Input: part model. Units: mm. Frame: model coordinates. A direction names the side the tool comes from. Coordinates: 2 decimals unless noted, no trailing zeros. Write each loop counter-clockwise with the first axis right and the second up, starting at its lowest first coordinate (ties: lowest second). Pieces come first, ordered by that corner, then holes. Notation, with made-up numbers: (49.5, 29) - (108.5, 29) arc R17 ccw to (108.5, 51) - close; hole circle Ø1 at (47, -15.75). An arc over 180 degrees is marked (long way). Use a Markdown table: item, result. Add a question column.
Q1. Section query C-C (z = 2.5). Give the number of separate pieces and of enclosed holes in the cut face, then the cut area to 3 significant figures.
Q2. Mould query, pull axis Y, two halves, no side actions, for faces 1 (the face through (72, 42, 0)), 2 (the face through (-95.47, -101.99, 1.57)), 3 (the face through (124.424, 125.214, 1.61)), 4 (the face through (-31.2, 16.3, 0.8)). Classes: released by +Y, released by -Y, zero draft, split by the parting line, or undercut.
Q3. Section query A-A (y = 39). Return the cut outline in (x, z) (1 decimal), then the cut area to 3 significant figures.
Q4. Pin query (flat end, axial travel): P1, Ø1.5, axis at x = 40, z = 2, coming from the -Y side; P2, Ø1, axis at y = 28.5, z = 2, coming from the -X side; P3, Ø1.5, axis at y = 15.5, z = 1, coming from the -X side. Return the tip coordinate at first contact, or that it passes through.
Q5. Set-up query: faces 5 (the face through (-67, -31, 1.588)), 6 (the face through (-122.77, -32.16, 1.61)). Return all of +Z, -Z, +X, -X, +Y, -Y with unobstructed straight access to the full face (end or side cutting, diameter ignored); none if empty.
Q6. Section query B-B (x = -116). Return the cut outline in (y, z) (1 decimal).
Q7. Section query D-D (y = -93.5). Return the cut outline in (x, z) (3 decimals).
Q8. Material intervals for probe 1 along X at (y, z) = (100, 0.7); probe 2 along Y at (x, z) = (60, 0.2); probe 3 along Y at (x, z) = (24.5, 2.35), sorted ascending. Write a range as from..to.
from build123d import *

# Parameters (mm, degrees)
BOSS_EXTRUDE1_DEPTH = 3.175
CUT_EXTRUDE3_DEPTH  = 1.5875
SKETCH3_R           = 9.525
CUT_EXTRUDE4_DEPTH  = 4.175
CUT_EXTRUDE5_DEPTH  = 4.175
FILLET1_R           = 50.8
SKETCH8_R           = 3.175
CUT_EXTRUDE7_DEPTH  = 4.175
SKETCH9_R           = 2.413
CUT_EXTRUDE8_DEPTH  = 4.175


with BuildPart() as part:
    # Sketch1 → Boss-Extrude1 (new body)
    with BuildSketch(Plane.XY):
        with BuildLine():
            Line((0, 139.7), (139.7, 139.7))
            Line((139.7, 139.7), (139.7, 0))
            ThreePointArc((139.7, 0), (-98.782817332, -98.782817332), (0, 139.7))
        make_face()
    extrude(amount=BOSS_EXTRUDE1_DEPTH)

    # Sketch2 → Cut-Extrude3 (cut)
    with BuildSketch(Plane(origin=(0, 0, 0), x_dir=(-1, 0, 0), z_dir=(0, 0, -1))):
        with BuildLine():
            ThreePointArc((-127.273929282, -57.597195461), (-126.611197849, -59.039771165), (-125.932116301, -60.474722685))
            Line((-125.932116301, -60.474722685), (-1.5875, -2.491875854))
            Line((-1.5875, -2.491875854), (-1.5875, -69.587590332))
            ThreePointArc((-1.5875, -69.587590332), (0, -69.162220989), (1.5875, -69.587590332))
            Line((1.5875, -69.587590332), (1.5875, -2.491875854))
            Line((1.5875, -2.491875854), (125.932116301, -60.474722685))
            ThreePointArc((125.932116301, -60.474722685), (126.611197849, -59.039771165), (127.273929282, -57.597195461))
            Line((127.273929282, -57.597195461), (3.756345013, 0))
            Line((3.756345013, 0), (55.328894815, 24.048674923))
            ThreePointArc((55.328894815, 24.048674923), (54.272472776, 25.307669683), (53.987081834, 26.926202147))
            Line((53.987081834, 26.926202147), (1.5875, 2.491875854))
            Line((1.5875, 2.491875854), (1.5875, 139.690979822))
            ThreePointArc((1.5875, 139.690979822), (0.793762813, 139.697744937), (0, 139.7))
            Line((0, 139.7), (-1.5875, 139.7))
            Line((-1.5875, 139.7), (-1.5875, 2.491875854))
            Line((-1.5875, 2.491875854), (-53.987081834, 26.926202147))
            ThreePointArc((-53.987081834, 26.926202147), (-54.272472776, 25.307669683), (-55.328894815, 24.048674923))
            Line((-55.328894815, 24.048674923), (-3.756345013, 0))
            Line((-3.756345013, 0), (-127.273929282, -57.597195461))
        make_face()
    extrude(amount=-CUT_EXTRUDE3_DEPTH, mode=Mode.SUBTRACT)

    # Sketch3 → Cut-Extrude4 (cut, through all)
    with BuildSketch(Plane.XY.offset(3.175)):
        Circle(SKETCH3_R)
    extrude(amount=-CUT_EXTRUDE4_DEPTH, mode=Mode.SUBTRACT)

    # Sketch2_4 → Cut-Extrude5 (cut, through all)
    with BuildSketch(Plane(origin=(0, 0, 0), x_dir=(-1, 0, 0), z_dir=(0, 0, -1))):
        with BuildLine():
            Line((-60.312918166, 26.37276318), (-55.328894815, 24.048674923))
            ThreePointArc((-55.328894815, 24.048674923), (-54.333740605, 25.183430817), (-53.975, 26.649482664))
            ThreePointArc((-53.975, 26.649482664), (-53.978021896, 26.787974218), (-53.987081834, 26.926202147))
            Line((-53.987081834, 26.926202147), (-58.971105185, 29.250290404))
            ThreePointArc((-58.971105185, 29.250290404), (-60.027527224, 27.991295645), (-60.312918166, 26.37276318))
        make_face()
        with BuildLine():
            ThreePointArc((-60.312918166, 26.37276318), (-58.491812981, 23.77195544), (-55.328894815, 24.048674923))
            Line((-55.328894815, 24.048674923), (-60.312918166, 26.37276318))
        make_face()
        with BuildLine():
            Line((-58.971105185, 29.250290404), (-53.987081834, 26.926202147))
            ThreePointArc((-53.987081834, 26.926202147), (-55.808187019, 29.527009887), (-58.971105185, 29.250290404))
        make_face()
        with BuildLine():
            ThreePointArc((53.987081834, 26.926202147), (54.272472776, 25.307669683), (55.328894815, 24.048674923))
            Line((55.328894815, 24.048674923), (60.312918166, 26.37276318))
            ThreePointArc((60.312918166, 26.37276318), (60.321978104, 26.510991109), (60.325, 26.649482664))
            ThreePointArc((60.325, 26.649482664), (59.966259395, 28.115534511), (58.971105185, 29.250290404))
            Line((58.971105185, 29.250290404), (53.987081834, 26.926202147))
        make_face()
        with BuildLine():
            ThreePointArc((58.971105185, 29.250290404), (55.808187019, 29.527009887), (53.987081834, 26.926202147))
            Line((53.987081834, 26.926202147), (58.971105185, 29.250290404))
        make_face()
        with BuildLine():
            Line((60.312918166, 26.37276318), (55.328894815, 24.048674923))
            ThreePointArc((55.328894815, 24.048674923), (58.491812981, 23.77195544), (60.312918166, 26.37276318))
        make_face()
        with BuildLine():
            Line((-1.5875, -75.086851646), (-1.5875, -69.587590332))
            ThreePointArc((-1.5875, -69.587590332), (-3.175, -72.337220989), (-1.5875, -75.086851646))
        make_face()
        with BuildLine():
            ThreePointArc((1.5875, -69.587590332), (0, -69.162220989), (-1.5875, -69.587590332))
            Line((-1.5875, -69.587590332), (-1.5875, -75.086851646))
            ThreePointArc((-1.5875, -75.086851646), (0, -75.512220989), (1.5875, -75.086851646))
            Line((1.5875, -75.086851646), (1.5875, -69.587590332))
        make_face()
        with BuildLine():
            ThreePointArc((3.175, -72.337220989), (2.749630657, -70.749720989), (1.5875, -69.587590332))
            Line((1.5875, -69.587590332), (1.5875, -75.086851646))
            ThreePointArc((1.5875, -75.086851646), (2.749630657, -73.924720989), (3.175, -72.337220989))
        make_face()
    extrude(amount=-CUT_EXTRUDE5_DEPTH, mode=Mode.SUBTRACT)

    # Fillet1
    fillet1_edges = [part.edges().sort_by_distance(p)[0] for p in [
        (139.7, 139.7, 1.5875),
    ]]
    fillet(fillet1_edges, radius=FILLET1_R)

    # Sketch8 → Cut-Extrude7 (cut, through all)
    with BuildSketch(Plane.XY.offset(3.175)):
        with Locations((25.0825, 101.6)):
            Circle(SKETCH8_R)
        with Locations((-25.0825, 101.6)):
            Circle(SKETCH8_R)
        with Locations((-25.0825, 127)):
            Circle(SKETCH8_R)
        with Locations((25.0825, 127)):
            Circle(SKETCH8_R)
        with Locations((102.681193713, -20.205550325)):
            Circle(SKETCH8_R)
        with Locations((125.701411504, -30.940054173)):
            Circle(SKETCH8_R)
        with Locations((81.480548613, -65.670480461)):
            Circle(SKETCH8_R)
        with Locations((104.500766404, -76.404984309)):
            Circle(SKETCH8_R)
        with Locations((-81.480548613, -65.670480461)):
            Circle(SKETCH8_R)
        with Locations((-104.500766404, -76.404984309)):
            Circle(SKETCH8_R)
        with Locations((-102.681193713, -20.205550325)):
            Circle(SKETCH8_R)
        with Locations((-125.701411504, -30.940054173)):
            Circle(SKETCH8_R)
    extrude(amount=-CUT_EXTRUDE7_DEPTH, mode=Mode.SUBTRACT)

    # Sketch9 → Cut-Extrude8 (cut, through all)
    with BuildSketch(Plane.XY.offset(3.175)):
        with Locations((90.4875, 104.775)):
            Circle(SKETCH9_R)
        with Locations((90.4875, 123.825)):
            Circle(SKETCH9_R)
        with Locations((100.6475, 104.775)):
            Circle(SKETCH9_R)
        with Locations((100.6475, 123.825)):
            Circle(SKETCH9_R)
        with Locations((63.8175, 104.775)):
            Circle(SKETCH9_R)
        with Locations((63.8175, 123.825)):
            Circle(SKETCH9_R)
    extrude(amount=-CUT_EXTRUDE8_DEPTH, mode=Mode.SUBTRACT)


solid = part.part
Values follow:
| question | item | result |
|---|---|---|
| 1 | separate pieces | 1 |
| 1 | enclosed holes | 22 |
| 1 | area | 64,100 mm2 |
| 2 | face 1 | zero draft |
| 2 | face 2 | split by the parting line |
| 2 | face 3 | released by +Y |
| 2 | face 4 | undercut |
| 3 | outline | (-134.1, 0) - (-1.6, 0) - (-1.6, 1.6) - (1.6, 1.6) - (1.6, 0) - (139.7, 0) - (139.7, 3.2) - (-134.1, 3.2) - close |
| 3 | area | 864 mm2 |
| 4 | P1 | y = -134.07 |
| 4 | P2 | x = -136.87 |
| 4 | P3 | x = -138.92 |
| 5 | face 5 | -Z |
| 5 | face 6 | +Z, -Z |
| 6 | outline | (-77.8, 0) - (-55.8, 0) - (-55.8, 1.6) - (-52.3, 1.6) - (-52.3, 0) - (77.8, 0) - (77.8, 3.2) - (-77.8, 3.2) - close |
| 7 | outline | (-103.797, 0) - (103.797, 0) - (103.797, 3.175) - (-103.797, 3.175) - close |
| 8 | probe 1 | -97.55..-27.82, -22.34..-1.59, 1.59..22.34, 27.82..138.47 |
| 8 | probe 2 | -126.16..-29.73, -26.23..25.25, 28.05..139.7 |
| 8 | probe 3 | -137.53..98.48, 104.72..123.88, 130.12..139.7 |
